from build123d import *

# Parameters (mm, degrees)
F0_W      = 80
F0_H      = 36
F1_DEPTH  = 1.6
F2_W      = 71.3
F2_H      = 26.3
F3_DEPTH  = 8.6
F4_W      = 64.5
F4_H      = 16.4
F5_DEPTH  = 0.5
F6_R      = 1.25
F7_DEPTH  = 1.601
F8_R      = 0.5
F9_DEPTH  = 1.601
F10_R     = 4.646555
F10_R_2   = 6.155936
F11_DEPTH = 3.3


with BuildPart() as f1:
    # F0 (on Front) → F1 (new body)
    with BuildSketch(Plane.XZ):
        with Locations((35.905228, 13.74974)):
            Rectangle(F0_W, F0_H)
    extrude(amount=F1_DEPTH)

    # F2 (on face) → F3 (join)
    with BuildSketch(Plane.XZ.offset(1.6)):
        with Locations((35.905228, 13.44974)):
            Rectangle(F2_W, F2_H)
    extrude(amount=F3_DEPTH)

    # F4 (on face) → F5 (cut)
    with BuildSketch(Plane.XZ.offset(10.2)):
        with Locations((35.905228, 13.44974)):
            Rectangle(F4_W, F4_H)
    extrude(amount=-F5_DEPTH, mode=Mode.SUBTRACT)

    # F6 (on face) → F7 (cut, through all)
    with BuildSketch(Plane.XZ.offset(1.6)):
        with Locations((-1.594772, 29.24974)):
            Circle(F6_R)
        with Locations((73.405228, 29.24974)):
            Circle(F6_R)
        with Locations((73.405228, -1.75026)):
            Circle(F6_R)
        with Locations((-1.594772, -1.75026)):
            Circle(F6_R)
    extrude(amount=-F7_DEPTH, mode=Mode.SUBTRACT)

    # F8 (on face) → F9 (cut, through all)
    with BuildSketch(Plane.XZ.offset(1.6)):
        with Locations((3.905228, 29.24974)):
            Circle(F8_R)
        with Locations((6.445228, 29.24974)):
            Circle(F8_R)
        with Locations((8.985228, 29.24974)):
            Circle(F8_R)
        with Locations((11.525228, 29.24974)):
            Circle(F8_R)
        with Locations((14.065228, 29.24974)):
            Circle(F8_R)
        with Locations((16.605228, 29.24974)):
            Circle(F8_R)
        with Locations((19.145228, 29.24974)):
            Circle(F8_R)
        with Locations((21.685228, 29.24974)):
            Circle(F8_R)
        with Locations((24.225228, 29.24974)):
            Circle(F8_R)
        with Locations((26.765228, 29.24974)):
            Circle(F8_R)
        with Locations((29.305228, 29.24974)):
            Circle(F8_R)
        with Locations((31.845228, 29.24974)):
            Circle(F8_R)
        with Locations((34.385228, 29.24974)):
            Circle(F8_R)
        with Locations((36.925228, 29.24974)):
            Circle(F8_R)
        with Locations((39.465228, 29.24974)):
            Circle(F8_R)
        with Locations((42.005228, 29.24974)):
            Circle(F8_R)
    extrude(amount=-F9_DEPTH, mode=Mode.SUBTRACT)

    # F10 (on face) → F11 (join)
    with BuildSketch(Plane(origin=(0, 0, 0), x_dir=(-1, 0, 0), z_dir=(0, 1, 0))):
        with Locations((-53.529158, 13.976525)):
            Circle(F10_R)
        with Locations((-19.490262, 14.239374)):
            Circle(F10_R_2)
    extrude(amount=F11_DEPTH)


solid = f1.part
The listing builds one solid part. Answer for the finished solid, in the listing's coordinates (mm). A direction names the side the tool comes from. Give positions to 0.01 mm unless a question says otherwise; leave off trailing zeros. Loops run counter-clockwise (first coordinate to the right, second up) from the corner with the lowest first, then second, coordinate; pieces in that order, holes last. Notation, with made-up numbers: (18, 83.25) - (48, 83.25) arc R5 ccw to (48, 87.25) - close; hole circle Ø6 at (-2.5, 80). An arc over 180 degrees is marked (long way). Use one line per item in the form item = value.
1. Section A-A on x = 65 is taken. Give the vertices of the cut face in (y, z).
Calculated:
outline = (-10.2, 0.3) - (-1.6, 0.3) - (-1.6, -4.25) - (0, -4.25) - (0, 31.75) - (-1.6, 31.75) - (-1.6, 26.6) - (-10.2, 26.6) - (-10.2, 21.65) - (-9.7, 21.65) - (-9.7, 5.25) - (-10.2, 5.25) - close
2. Given pin 1 Ø2 at (x, z) = (54, 16) entering from -Y; pin 2 Ø4 at (x, z) = (-1.59, 29.25) entering from -Y; pin 3 Ø7 at (y, z) = (-7.5, 19) entering from +X; pin 4 Ø12 at (x, z) = (23.5, 8.5) entering from -Y, each flat-ended and moving along its own axis, determine where each tip first touches the part or whether it passes through.
Calculated:
pin_1 = -9.7
pin_2 = -1.6
pin_3 = 71.56
pin_4 = -10.2
3. Which of the six approach directions +Z, -Z, +X, -X, +Y, -Y give full straight-line access (tool end or side, diameter ignored) to faces 1 (the face through (71.555, -6, 13)), 2 (the face through (35, -9.7, 14)), 3 (the face through (35, -6, 26.6)), 4 (the face through (24.375, 1.627, 10.494))?
Calculated:
face_1 = +Z, -Z, +X, -Y
face_2 = -Y
face_3 = +Z, +X, -X, -Y
face_4 = +Y
4. Section C-C on z = 17 is taken. Give the vertices of the cut face in (x, y).
Calculated:
outline = (-4.09, -1.6) - (0.26, -1.6) - (0.26, -10.2) - (3.66, -10.2) - (3.66, -9.7) - (68.16, -9.7) - (68.16, -10.2) - (71.56, -10.2) - (71.56, -1.6) - (75.91, -1.6) - (75.91, 0) - (57.06, 0) - (57.06, 3.3) - (50, 3.3) - (50, 0) - (24.99, 0) - (24.99, 3.3) - (13.99, 3.3) - (13.99, 0) - (-4.09, 0) - close
5. Section B-B on y = 1.5 is taken. Give the vertices of the cut face in (x, z).
Calculated:
outline = circle Ø12.31 at (19.49, 14.24); circle Ø9.29 at (53.53, 13.98)
6. Section D-D on y = -2.5 is taken. Give the vertices of the cut face in (x, z), then the cut area to 3 significant figures.
Calculated:
outline = (0.26, 0.3) - (71.56, 0.3) - (71.56, 26.6) - (0.26, 26.6) - close
area = 1,880 mm^2
7. Find the intervals of material crossed by line 1 along X through (y, z) = (0.25, 14); line 2 along X through (y, z) = (-1.5, 28.5); line 3 along Z through (x, y) = (72.5, -1.25), in increasing order. Write a range as [from, to].
Calculated:
line_1 = [13.34, 25.64], [48.88, 58.18]
line_2 = [-4.09, -2.59], [-0.59, 72.41], [74.41, 75.91]
line_3 = [-4.25, -2.61], [-0.89, 28.39], [30.11, 31.75]
8. The mould has two halves that part along X. Classify faces 5 (the face through (74.598, -0.811, -1.375)), 6 (the face through (35, -1, 31.75)), 7 (the face through (0.255, -6, 13)): pulls with the +X half, pulls with the -X half, needs draft (parallel to the pull), parting line crosses it, or undercut.
Calculated:
face_5 = undercut
face_6 = needs draft
face_7 = pulls with the -X half
